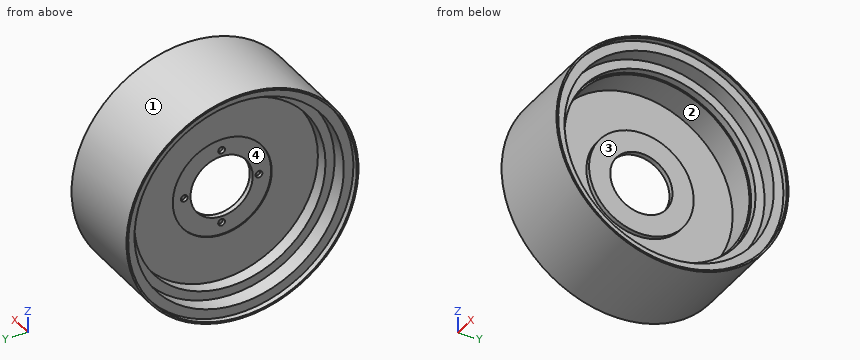
```python
from build123d import *

# Parameters (mm, degrees)
F2_R            = 6
F3_DEPTH        = 6
F3_COPIES_COUNT = 4


# Not quite as in the source:
# - a pattern or mirror of a feature is missing from the dataset's text; its kind, count and spacing are read off the source's solid


with BuildPart() as f1:
    # F0 (on Front) → F1 (revolve)
    with BuildSketch(Plane.XZ):
        Polygon((166, 205), (0, 205), (0, 202), (10, 202), (10, 185), (38, 185), (38, 169), (61, 169), (61, 87.5), (63, 87.5), (63, 55), (72, 55), (72, 92.5), (64, 92.5), (64, 166), (115, 166), (115, 169), (128, 169), (128, 185), (156, 185), (156, 202), (166, 202), align=None)
    revolve(axis=Axis((83, 0, 0), (1, 0, 0)))

    # F2 (on face) → F3 (cut)
    with BuildSketch(Plane(origin=(63, 0, 0), x_dir=(0, -1, 0), z_dir=(-1, 0, 0))):
        with Locations((0, 66)):
            Circle(F2_R)
    f3 = extrude(amount=-F3_DEPTH, mode=Mode.SUBTRACT)

    # F3_copies: F3 ×4 about axis
    f3_copies_axis = Axis((0, 0, 0), (1, 0, 0))
    for i in range(1, F3_COPIES_COUNT):
        add(f3.rotate(f3_copies_axis, i * 360 / F3_COPIES_COUNT), mode=Mode.SUBTRACT)


solid = f1.part
```
Check sheet for the modelled part. Datum: model origin and axes. Units: mm. Face numbers are marked on the shaded views. A direction names the side the tool comes from. Coordinates: 2 decimals unless noted, no trailing zeros. Write each loop counter-clockwise with the first axis right and the second up, starting at its lowest first coordinate (ties: lowest second). Pieces come first, ordered by that corner, then holes. Notation, with made-up numbers: (-28.5, -34) -> (17.5, -34) arc R22 ccw to (17.5, 1) -> close; hole circle Ø6 at (50, 64.25). An arc over 180 degrees is marked (long way). Use a Markdown table: item, result.
1. Go/stop test with flat-tipped pins: pin 1 Ø6 at (y, z) = (-54, -143) entering from -X; pin 2 Ø2 at (y, z) = (-96.5, 141) entering from +X; pin 3 Ø4 at (x, y) = (88, 50) entering from +Z. Record where each tip stops, or that it passes through.
Reported:
| item | result |
|---|---|
| pin 1 | stops at x = 61 |
| pin 2 | stops at x = 128 |
| pin 3 | stops at z = 199.3 |
2. Tool access check on the marked faces 3 and 4. Record the directions out of +Z, -Z, +X, -X, +Y, -Y that give a thin tool (end or side, any length) a straight path to the whole face; none if there is none.
Reported:
| item | result |
|---|---|
| face 3 | +X |
| face 4 | -X |
3. Sectioned sample at B-B (y = 174). Enter the section's corners in (x, z).
Reported:
| item | result |
|---|---|
| outline | (0, -108.39) -> (166, -108.39) -> (166, -102.61) -> (156, -102.61) -> (156, -62.84) -> (128, -62.84) -> (128, 62.84) -> (156, 62.84) -> (156, 102.61) -> (166, 102.61) -> (166, 108.39) -> (0, 108.39) -> (0, 102.61) -> (10, 102.61) -> (10, 62.84) -> (38, 62.84) -> (38, -62.84) -> (10, -62.84) -> (10, -102.61) -> (0, -102.61) -> close |
4. Sectioned sample at A-A (x = 85). Enter the section's corners in (y, z).
Reported:
| item | result |
|---|---|
| outline | circle Ø410 at (0, 0); hole circle Ø332 at (0, 0) |
5. Release check for a two-part mould opening along Y. For the marked faces 1 and 2 record: pulls with the +Y half, pulls with the -Y half, needs draft (parallel to the pull), parting line crosses it, or undercut.
Reported:
| item | result |
|---|---|
| face 1 | parting line crosses it |
| face 2 | undercut |
6. Scan lines: line 1 along Y through (x, z) = (80, 0); line 2 along Z through (x, y) = (61.65, 0). Record each from-to range of solid material in increasing order.
Reported:
| item | result |
|---|---|
| line 1 | y = -205 to -166, 166 to 205 |
| line 2 | z = -205 to -87.5, 87.5 to 205 |
